```python
from build123d import *

# Parameters (mm, degrees)
F1_DEPTH = 12
F2_DEPTH = 4


with BuildPart() as f1:
    # F0 (on Top) → F1 (new body)
    with BuildSketch(Plane.XY):
        with BuildLine():
            ThreePointArc((-14.2014003754, -5.5286388661), (-15.3436839287, -2.7709224195), (-18.1014003754, -1.6286388661))
            Line((-18.1014003754, -1.6286388661), (-18.1014003754, -9.4286388661))
            ThreePointArc((-18.1014003754, -9.4286388661), (-15.3436839287, -8.2863553127), (-14.2014003754, -5.5286388661))
        make_face()
        with BuildLine():
            Line((-18.1014003754, -9.4286388661), (-18.1014003754, -1.6286388661))
            ThreePointArc((-18.1014003754, -1.6286388661), (-22.0014003754, -5.5286388661), (-18.1014003754, -9.4286388661))
        make_face()
    extrude(amount=F1_DEPTH)



with BuildPart() as f1b:
    # F0 (on Top) → F1, piece 2 (new body)
    with BuildSketch(Plane.XY):
        with BuildLine():
            ThreePointArc((24.1485996246, -5.5286388661), (23.0063160713, -2.7709224195), (20.2485996246, -1.6286388661))
            Line((20.2485996246, -1.6286388661), (20.2485996246, -9.4286388661))
            ThreePointArc((20.2485996246, -9.4286388661), (23.0063160713, -8.2863553127), (24.1485996246, -5.5286388661))
        make_face()
        with BuildLine():
            Line((20.2485996246, -9.4286388661), (20.2485996246, -1.6286388661))
            ThreePointArc((20.2485996246, -1.6286388661), (16.3485996246, -5.5286388661), (20.2485996246, -9.4286388661))
        make_face()
    extrude(amount=F1_DEPTH)


with BuildPart() as f1_1:
    add(f1.part)

    add(f1b.part)  # F2 merges F1b
    # F0 (on Top) → F2 (join)
    with BuildSketch(Plane.XY):
        with BuildLine():
            Line((20.2485996246, -0.5286388661), (-18.1014003754, -0.5286388661))
            Line((-18.1014003754, -0.5286388661), (-18.1014003754, -1.6286388661))
            ThreePointArc((-18.1014003754, -1.6286388661), (-15.3436839287, -2.7709224195), (-14.2014003754, -5.5286388661))
            ThreePointArc((-14.2014003754, -5.5286388661), (-15.3436839287, -8.2863553127), (-18.1014003754, -9.4286388661))
            Line((-18.1014003754, -9.4286388661), (-18.1014003754, -10.5286388661))
            Line((-18.1014003754, -10.5286388661), (20.2485996246, -10.5286388661))
            Line((20.2485996246, -10.5286388661), (20.2485996246, -9.4286388661))
            ThreePointArc((20.2485996246, -9.4286388661), (16.3485996246, -5.5286388661), (20.2485996246, -1.6286388661))
            Line((20.2485996246, -1.6286388661), (20.2485996246, -0.5286388661))
        make_face()
    extrude(amount=F2_DEPTH)


solid = f1_1.part
```
Here's how the part is built. I have some questions about the finished solid (model axes, mm). A direction names the side the tool comes from. Round coordinates to 2 decimals unless told otherwise and drop trailing zeros. Loops run counter-clockwise (first coordinate to the right, second up) from the corner with the lowest first, then second, coordinate; pieces in that order, holes last. Notation, with made-up numbers: (81, 1.25) -> (99, 1.25) arc R23 cw to (99, 22.25) -> close; hole circle Ø2 at (68, -12.75). An arc over 180 degrees is marked (long way). Answer as CSV lines item,"result".
1. If we section it at A-A on z = 2: Please give me the cut outline in (x, y), plus the area to 3 significant figures.
Final values:
outline,"(-18.1, -10.53) -> (20.25, -10.53) -> (20.25, -9.43) arc R3.9 ccw to (20.25, -1.63) -> (20.25, -0.53) -> (-18.1, -0.53) -> (-18.1, -1.63) arc R3.9 ccw to (-18.1, -9.43) -> close"
area,"431 mm^2"
2. If we section it at C-C on x = -4.5: Please give me the cut outline in (y, z), plus the area to 3 significant figures.
Final values:
outline,"(-10.53, 0) -> (-0.53, 0) -> (-0.53, 4) -> (-10.53, 4) -> close"
area,"40.0 mm^2"
3. Which directions (+Z, -Z, +X, -X, +Y, -Y) give clear straight access to the entire face, cutting with the end or side of a thin tool? Please do faces 1 (the face through (20.249, -10, 2)), 2 (the face through (-18.101, -1, 2)), 3 (the face through (1, -5, 0)).
Final values:
face 1,"+Z, -Z, +X, -Y"
face 2,"+Z, -Z, -X, +Y"
face 3,"-Z, +X, -X, +Y, -Y"
4. Thinking about a two-plate mould opening in X: for faces 4 (the face through (-18.101, -10, 2)), 5 (the face through (20.249, -1, 2)), 6 (the face through (1, -5, 4)), which applies, released by +X, released by -X, zero draft, split by the parting line, or undercut?
Final values:
face 4,"released by -X"
face 5,"released by +X"
face 6,"undercut"
5. If I drill on L1, parallel to Z at x = -2.5, y = -10; L2, parallel to X at y = -2.75, z = 5; L3, parallel to X at y = -9, z = 10, over which ranges is the centre line in solid material (lowest first)?
Final values:
L1,"z = 0 to 4"
L2,"x = -20.84 to -15.36, 17.51 to 22.99"
L3,"x = -19.88 to -16.32, 18.47 to 22.03"
6. If we section it at B-B on z = 6.5: Please give me the cut outline in (x, y).
Final values:
outline,"circle Ø7.8 at (-18.1, -5.53); circle Ø7.8 at (20.25, -5.53)"
7. For pin 1 (0.9 mm diameter, centred on y = -1, z = 1.5, fed in from -X); pin 2 (5 mm diameter, centred on x = 9.5, y = -4.5, fed in from +Z); pin 3 (1.5 mm diameter, centred on y = -3.5, z = 10.5, fed in from +X), each with a flat end and sliding along its axis, tell me the tip position at first contact or that it passes through.
Final values:
pin 1,"stops at x = -18.1"
pin 2,"stops at z = 4"
pin 3,"stops at x = 23.93"
8. If we section it at D-D on y = -3: Please give me the cut outline in (x, z), plus the area to 3 significant figures.
Final values:
outline,"(-21.07, 0) -> (23.22, 0) -> (23.22, 12) -> (17.28, 12) -> (17.28, 4) -> (-15.13, 4) -> (-15.13, 12) -> (-21.07, 12) -> close"
area,"272 mm^2"
